```python
from build123d import *

# Parameters (mm, degrees)
SKETCH_1_W          = 45
SKETCH_1_H          = 43
EXTRUDE_1_DEPTH     = 23
SHELL_1_T           = -1.5
SKETCH_2_R          = 1.5
CUT_EXTRUDE_1_DEPTH = 54.7052139
FILLET_1_R          = 1.5
FILLET_2_R          = 2


with BuildPart() as part:
    # 草图1 → 凸台-拉伸1 (new body)
    with BuildSketch(Plane(origin=(0, 0, 0), x_dir=(1, 0, 0), z_dir=(0, 1, 0))):
        Rectangle(SKETCH_1_W, SKETCH_1_H)
    extrude(amount=EXTRUDE_1_DEPTH)

    # 抽壳1
    shell_1_openings = [part.faces().sort_by_distance(p)[0] for p in [
        (0, 0, 0),
        (22.5, 11.5, 0),
        (-22.5, 11.5, 0),
    ]]
    offset(amount=SHELL_1_T, openings=shell_1_openings, kind=Kind.INTERSECTION)

    # 草图2 → 切除-拉伸1 (cut, through all)
    with BuildSketch(Plane.XY.offset(21.5)):
        with Locations((-17.5, 11.5)):
            Circle(SKETCH_2_R)
        with Locations((17.5, 11.5)):
            Circle(SKETCH_2_R)
    extrude(amount=-CUT_EXTRUDE_1_DEPTH, mode=Mode.SUBTRACT)

    # 圆角1
    fillet_1_edges = [part.edges().sort_by_distance(p)[0] for p in [
        (0, 23, -21.5),
        (0, 23, 21.5),
    ]]
    fillet(fillet_1_edges, radius=FILLET_1_R)

    # 圆角2
    fillet_2_edges = [part.edges().sort_by_distance(p)[0] for p in [
        (-22.5, 0, 20.75),
        (22.5, 0, -20.75),
        (22.5, 0, 20.75),
        (-22.5, 0, -20.75),
    ]]
    fillet(fillet_2_edges, radius=FILLET_2_R)


solid = part.part
```
Could you check a few things on this model? Use its own coordinates, in mm. A direction names the side the tool comes from. Coordinates: 2 decimals unless noted, no trailing zeros. Order: outer loops, then holes, each group sorted by start corner. A loop starts at its lowest first (then second) coordinate and runs counter-clockwise, first axis right, second up. Notation, with made-up numbers: M -25,-9 L 6,-9 A23 ccw 6,4 Z; hole C 3,22 d9. An arc over 180 degrees is marked long. Use a Markdown table: item, result. Add a question column.
Q1. Which directions (+Z, -Z, +X, -X, +Y, -Y) give clear straight access to the entire face, cutting with the end or side of a thin tool? Please do faces 5 (the flat face through (0, 23, 0)), 6 (the flat face through (0, 21.5, 0)).
Q2. If I drill on L1, parallel to Z at x = 0, y = 12; L2, parallel to Y at x = -5, z = -9.5; L3, parallel to Y at x = -17.5, z = 20.8, over which ranges is the centre line in solid material (lowest first)?
Q3. We'd pull the mould along Y, two halves only. Please class faces 1 (the cylindrical face through (16, 11.57, -20.74)), 2 (the cylindrical face through (-21.93, 0.6, 20.74)), 3 (the flat face through (0, 11, -20)), 4 (the cylindrical face through (0.32, 22.57, -21.05)): pulls with the +Y half, pulls with the -Y half, needs draft (parallel to the pull), parting line crosses it, or undercut.
Q4. I'm going to push a flat-ended pin straight in: pin 1 (6 mm diameter, centred on x = -14, z = 12, fed in from -Y). Where does the tip first touch, or does it pass through?
Q5. I want a section at C-C on y = 11.5. List the corners of the cut face in (x, z) for me.
Q6. I want a section at B-B on x = 17.5. List the corners of the cut face in (y, z) for me, then the cut area to 3 significant figures.
Q7. I want a section at A-A on y = 16. List the corners of the cut face in (x, z) for me, then the cut area to 3 significant figures.
Q8. I want a section at D-D on x = 3. List the corners of the cut face in (y, z) for me.
Checked values:
| question | item | result |
|---|---|---|
| 1 | face 5 | +Z, -Z, +X, -X, +Y |
| 1 | face 6 | +X, -X, -Y |
| 2 | L1 | -21.5 to -20, 20 to 21.5 |
| 2 | L2 | 21.5 to 23 |
| 2 | L3 | 0 to 10, 13 to 22.77 |
| 3 | face 1 | undercut |
| 3 | face 2 | pulls with the -Y half |
| 3 | face 3 | needs draft |
| 3 | face 4 | pulls with the +Y half |
| 4 | pin 1 | y = 21.5 |
| 5 | outline | M -22.5,-21.5 L -19,-21.5 L -19,-20 L -22.5,-20 Z; M -22.5,20 L -19,20 L -19,21.5 L -22.5,21.5 Z; M -16,-21.5 L 16,-21.5 L 16,-20 L -16,-20 Z; M -16,20 L 16,20 L 16,21.5 L -16,21.5 Z; M 19,-21.5 L 22.5,-21.5 L 22.5,-20 L 19,-20 Z; M 19,20 L 22.5,20 L 22.5,21.5 L 19,21.5 Z |
| 6 | outline | M 0,-21.5 L 10,-21.5 L 10,-20 L 0,-20 Z; M 0,20 L 10,20 L 10,21.5 L 0,21.5 Z; M 13,-21.5 L 21.5,-21.5 A1.5 ccw 23,-20 L 23,20 A1.5 ccw 21.5,21.5 L 13,21.5 L 13,20 L 21.5,20 L 21.5,-20 L 13,-20 Z |
| 6 | area | 119 mm² |
| 7 | outline | M -22.5,-21.5 L 22.5,-21.5 L 22.5,-20 L -22.5,-20 Z; M -22.5,20 L 22.5,20 L 22.5,21.5 L -22.5,21.5 Z |
| 7 | area | 135 mm² |
| 8 | outline | M 0,-21.5 L 21.5,-21.5 A1.5 ccw 23,-20 L 23,20 A1.5 ccw 21.5,21.5 L 0,21.5 L 0,20 L 21.5,20 L 21.5,-20 L 0,-20 Z |
